Geometry check sheet. Reference: the model listing, model coordinates, mm. Round coordinates to 2 decimals unless told otherwise and drop trailing zeros. Order: outer loops, then holes, each group sorted by start corner. A loop starts at its lowest first (then second) coordinate and runs counter-clockwise, first axis right, second up. Notation, with made-up numbers: (21, 84) - (39, 84) arc R22 cw to (39, 101) - close; hole circle Ø4 at (-12.75, 15.5). An arc over 180 degrees is marked (long way). One line per question, with ' | ' between items. Start each with the question number.
Q1. Sectioned sample at D-D, the plane x = 7.5. Enter the section's corners in (y, z) (3 decimals).
Q2. Sectioned sample at B-B, the plane y = 0.4. Enter the section's corners in (x, z).
Q3. Mould release check, pull along X, two halves, no side actions. Record for faces 1 (the face through (0, 1, 0)), 2 (the face through (0.379, 0.493, -5.658)), 3 (the face through (-1.617, 0.493, 8.036)), 4 (the face through (-0.056, 0.493, -10.616)): +X half, -X half, draft (parallel to the pull), parting line (faces both ways), or undercut.
Q4. Sectioned sample at A-A, the plane x = 0. Enter the section's corners in (y, z).
Q5. Material ranges on line 1 along Z through (x, y) = (-0.75, 0.6); line 2 along Z through (x, y) = (1, 0.75); line 3 along X through (y, z) = (0.35, 6), recorded low to high.
Q6. Sectioned sample at C-C, the plane z = 3. Enter the section's corners in (x, y), then the cut area to 3 significant figures.
Autodesk Inventor part; units mm, degrees
ref_plane "YZ Plane" through (0, 0, 0) normal (1, 0, 0) x (0, 1, 0)
ref_plane "XZ Plane" through (0, 0, 0) normal (0, 1, 0) x (-1, 0, 0)
ref_plane "XY Plane" through (0, 0, 0) normal (0, 0, 1) x (1, 0, 0)
sketch "Sketch1" plane through (0, 0, 0) normal (0, 1, 0) x (-1, 0, 0)
  circle A0 centre (0, 7.366) radius 1.75
  circle A1 centre (0, -7.366) radius 1.75
  arc A2 (3.0588, -8.4643) -> (3.0588, 8.4643) centre (0, 0) ccw
  arc A3 (-3.0588, 8.4643) -> (-3.0588, -8.4643) centre (0, 0) ccw
  arc A4 (3.0588, 8.4643) -> (-3.0588, 8.4643) centre (0, 7.366) ccw
  arc A5 (-3.0588, -8.4643) -> (3.0588, -8.4643) centre (0, -7.366) ccw
  point P0 (9, 0)
extrude "Extrusion1" add sketch "Sketch1" along normal blind 1
properties part number "Ball Caster Spacer"
Determined:
1) outline: (0, -4.975) - (1, -4.975) - (1, 4.975) - (0, 4.975) - close
2) outline: (-3.06, -8.46) arc R3.25 ccw to (3.06, -8.46) arc R9 ccw to (3.06, 8.46) arc R3.25 ccw to (-3.06, 8.46) arc R9 ccw to start; hole circle Ø3.5 at (0, -7.37); hole circle Ø3.5 at (0, 7.37)
3) face 1: draft | face 2: undercut | face 3: undercut | face 4: parting line
4) outline: (0, -10.62) - (1, -10.62) - (1, -9.12) - (0, -9.12) - close; (0, -5.62) - (1, -5.62) - (1, 5.62) - (0, 5.62) - close; (0, 9.12) - (1, 9.12) - (1, 10.62) - (0, 10.62) - close
5) line 1: z = -10.53 to -8.95, -5.78 to 5.78, 8.95 to 10.53 | line 2: z = -10.46 to -8.8, -5.93 to 5.93, 8.8 to 10.46 | line 3: x = -6.71 to -1.09, 1.09 to 6.71
6) outline: (-8.49, 0) - (8.49, 0) - (8.49, 1) - (-8.49, 1) - close | area: 17.0 mm2
